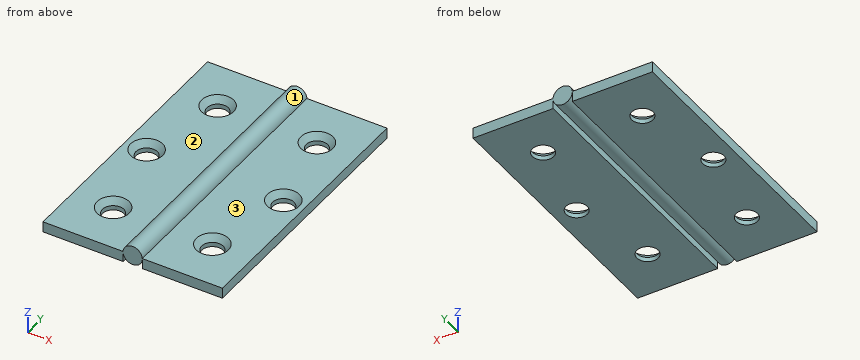
```python
from build123d import *

# Parameters (mm, degrees)
F0_W           = 19.05
F0_H           = 63.5
F1_DEPTH       = 2.54
F3_DEPTH       = 63.5
F5_D           = 5.08
F5_CSINK_D     = 7.62
F5_CSINK_ANGLE = 82


with BuildPart() as f1:
    # F0 (on Top) → F1 (new body)
    with BuildSketch(Plane.XY):
        with Locations((-45.6372228205, 17.373234883)):
            Rectangle(F0_W, F0_H)
    extrude(amount=F1_DEPTH)



with BuildPart() as f1b:
    # F0 (on Top) → F1, piece 2 (new body)
    with BuildSketch(Plane.XY):
        with Locations((-22.0152228205, 17.373234883)):
            Rectangle(F0_W, F0_H)
    extrude(amount=F1_DEPTH)


with BuildPart() as f1_1:
    add(f1.part)

    add(f1b.part)  # F3 merges F1b
    # F2 (on face) → F3 (join)
    with BuildSketch(Plane(origin=(0, 49.123234883, 0), x_dir=(-1, 0, 0), z_dir=(0, 1, 0))):
        with BuildLine():
            Line((31.5402228205, 2.54), (31.5402228205, 2.2870220252))
            ThreePointArc((31.5402228205, 2.2870220252), (33.8262228205, 0.1240142417), (36.1122228205, 2.2870220252))
            Line((36.1122228205, 2.2870220252), (36.1122228205, 2.54))
            ThreePointArc((36.1122228205, 2.54), (33.8262228205, 4.7030077835), (31.5402228205, 2.54))
        make_face()
    extrude(amount=-F3_DEPTH)

    # F5 (through all)
    with Locations(Plane.XY.offset(2.54)):
        with Locations((-45.6372228205, -2.7734471262), (-22.0152228205, -2.7734471262), (-17.5702228205, 17.373234883), (-50.0948168337, 17.373234883), (-45.6372228205, 37.5199168921), (-22.0152228205, 37.5199168921)):
            CounterSinkHole(F5_D / 2, F5_CSINK_D / 2, counter_sink_angle=F5_CSINK_ANGLE)


solid = f1_1.part
```
The listing builds one solid part. Answer for the finished solid, in the listing's coordinates (mm). Face numbers are marked on the shaded views. A direction names the side the tool comes from. Coordinates: 2 decimals unless noted, no trailing zeros. Write each loop counter-clockwise with the first axis right and the second up, starting at its lowest first coordinate (ties: lowest second). Pieces come first, ordered by that corner, then holes. Notation, with made-up numbers: (-4, 89.5) - (53, 89.5) arc R22 cw to (53, 119.5) - close; hole circle Ø10 at (30, 70). An arc over 180 degrees is marked (long way). Return JSON: item names as keys, results as strings. Group by question number.
1. A cutting plane is placed at A-A, the plane y = 24. Determine the outline of the cut face in (x, z).
2. A cutting plane is placed at C-C, the plane y = 36. Give the number of separate pieces and of enclosed holes in the cut face, plus the area to 3 significant figures.
3. Which of the six approach directions +Z, -Z, +X, -X, +Y, -Y give full straight-line access (tool end or side, diameter ignored) to the marked faces 1, 2 and 3?
4. A cutting plane is placed at D-D, the plane z = 4.05. Determine the outline of the cut face in (x, y), plus the area to 3 significant figures.
5. A cutting plane is placed at B-B, the plane x = -30.5. Determine the outline of the cut face in (y, z).
6. Straight lines are drawn through the part: L1, parallel to Y at x = -45.5, z = 0.2; L2, parallel to X at y = 46, z = 1.2; L3, parallel to X at y = -8.5, z = 0.6. For each, find the intervals that lie inside material, in ascending order.
7. Given pin 1 (6.5 mm diameter, centred on x = -50.09, y = 17.37, fed in from +Z); pin 2 (21 mm diameter, centred on x = -20, y = 23, fed in from +Z); pin 3 (4.5 mm diameter, centred on x = -22.02, y = -2.77, fed in from -Z); pin 4 (1.5 mm diameter, centred on y = 6.5, z = 4, fed in from +X) (3 decimals), each flat-ended and moving along its own axis, determine where each tip first touches the part or whether it passes through.
Ans:
{
 "1": {"outline": "(-55.16, 0) - (-36.11, 0) - (-36.11, 2.29) arc R2.29 ccw to (-31.54, 2.29) - (-31.54, 0) - (-12.49, 0) - (-12.49, 2.54) - (-31.54, 2.54) arc R2.29 ccw to (-36.11, 2.54) - (-55.16, 2.54) - close"},
 "2": {"separate pieces": "3", "enclosed holes": "0", "area": "88.2 mm²"},
 "3": {"face 1": "+Z, +Y, -Y", "face 2": "+Z, -X, +Y, -Y", "face 3": "+Z, +X, +Y, -Y"},
 "4": {"outline": "(-35.43, -14.38) - (-32.23, -14.38) - (-32.23, 49.12) - (-35.43, 49.12) - close", "area": "203 mm²"},
 "5": {"outline": "(-14.38, 0) - (49.12, 0) - (49.12, 2.54) - (-14.38, 2.54) - close"},
 "6": {"L1": "-14.38 to -5.31, -0.24 to 34.98, 40.06 to 49.12", "L2": "-55.16 to -36.11, -35.77 to -31.88, -31.54 to -12.49", "L3": "-55.16 to -36.11, -35.22 to -32.43, -31.54 to -12.49"},
 "7": {"pin 1": "z = 1.9", "pin 2": "z = 2.54", "pin 3": "through", "pin 4": "x = -31.695"}
}
